Input: part model. Units: mm. Frame: model coordinates. Face numbers are marked on the shaded views. A direction names the side the tool comes from. Coordinates: 2 decimals unless noted, no trailing zeros. Write each loop counter-clockwise with the first axis right and the second up, starting at its lowest first coordinate (ties: lowest second). Pieces come first, ordered by that corner, then holes.
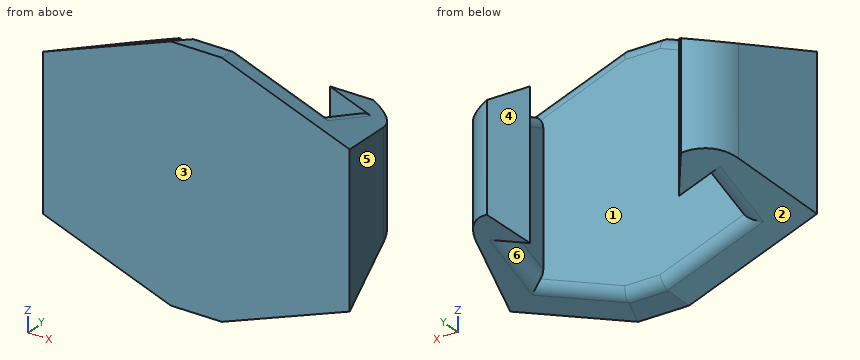
from build123d import *

# Parameters (mm, degrees)
EXTRUDE_1_DEPTH          = 20
CUT_EXTRUDE_1_DEPTH      = 26.52668646
CUT_EXTRUDE_1_DEPTH_BACK = 26.52668646
FILLET_1_R               = 4
CHAMFER_1_SIZE           = 10
CHAMFER_1_SIZE_2         = 3.739269956
FILLET_2_R               = 1


with BuildPart() as part:
    # 草圖2 → 填料-伸長1 (new body)
    with BuildSketch(Plane.XY):
        Polygon((-8.195537152, 3.678491207), (-10.195537152, 3.678491207), (-10.195537152, -0.821508793), (5.804462848, -0.821508793), (5.804462848, 3.678491207), (3.804462848, 3.678491207), (5.618474025, 6.178491207), (7.618474025, 6.178491207), (10.163991353, -3.321508793), (-14.609516351, -3.321508793), (-12.063999023, 6.178491207), (-10.063999023, 6.178491207), align=None)
    extrude(amount=EXTRUDE_1_DEPTH)

    # 草圖3 → 除料-伸長1 (cut, two sides: drawn at the far end of the back side and taken through both)
    with BuildSketch(Plane(origin=(0, 0, 0), x_dir=(0, 0, -1), z_dir=(1, 0, 0)).offset(-CUT_EXTRUDE_1_DEPTH_BACK)):
        Polygon((-20, -3.321508793), (-17.454482672, 6.178491207), (-20, 6.178491207), align=None)
        Polygon((0, 6.178491207), (-2.545517328, 6.178491207), (0, -3.321508793), align=None)
    extrude(amount=CUT_EXTRUDE_1_DEPTH + CUT_EXTRUDE_1_DEPTH_BACK, mode=Mode.SUBTRACT)

    # 圓角1
    # the kernel refuses this fillet: 4 mm, written as the material it takes off along each edge
    with BuildSketch(Plane(origin=(7.618474025, 6.178491207, -4.720017408), x_dir=(-1, 0, 0), z_dir=(0, 0, 1))) as fillet_1_piece_1:
        with BuildLine():
            CenterArc((3.1115198, 3.842463238), FILLET_1_R, 195, 58.866285833)
            Line((-0.752183505, 2.807187057), (-0.829457571, 2.786481534))
            Line((-0.829457571, 2.786481534), (-0.077274066, -0.020705524))
            Line((-0.077274066, -0.020705524), (0, -0.08))
            ThreePointArc((0, -0.08), (1, -0.08), (1.977769604, -0.076849265))
            Line((1.977769604, -0.076849265), (2, 0))
        make_face()
    extrude(amount=29.440034816, mode=Mode.SUBTRACT)
    with BuildSketch(Plane(origin=(-12.063999023, 6.178491207, -4.720017408), x_dir=(1, 0, 0), z_dir=(0, 0, 1))) as fillet_1_piece_2:
        with BuildLine():
            CenterArc((3.1115198, -3.842463238), FILLET_1_R, 106.133714167, 58.866285833)
            Line((-0.752183505, -2.807187057), (-0.829457571, -2.786481534))
            Line((-0.829457571, -2.786481534), (-0.077274066, 0.020705524))
            Line((-0.077274066, 0.020705524), (0, 0.08))
            ThreePointArc((0, 0.08), (1, 0.08), (1.977769604, 0.076849265))
            Line((1.977769604, 0.076849265), (2, 0))
        make_face()
    extrude(amount=29.440034816, mode=Mode.SUBTRACT)

    # 導角1
    # the kernel refuses this chamfer: 10, 3.739269956 mm, written as the material it takes off along each edge
    with BuildSketch(Plane(origin=(16.664078496, -27.580164265, -6.500087143), x_dir=(-0.9680162049238082, -0.23859176587740763, -0.07757961240176374), z_dir=(-0.25056280708573614, 0.9351131265310298, 0.25056280708572526)), Plane(origin=(-6.316095385, 27.629959622, 8.293420966), x_dir=(0.9680162049238085, -0.23859176587740732, -0.0775796124017635), z_dir=(-0.2505628070857358, -0.93511312653103, -0.2505628070857253)), Plane(origin=(-21.109603495, -27.580164265, 26.500087143), x_dir=(0.9680162049238082, -0.23859176587740735, 0.07757961240176349), z_dir=(0.25056280708573586, 0.9351131265310301, -0.2505628070857251)), Plane(origin=(1.870570387, 27.629959622, 11.706579034), x_dir=(-0.9680162049238082, -0.23859176587740777, 0.07757961240176336), z_dir=(0.25056280708573614, -0.93511312653103, 0.25056280708572504))) as chamfer_1_piece_1:
        Polygon((CHAMFER_1_SIZE * 0.999913086528, CHAMFER_1_SIZE * 0.0131840581986), (-CHAMFER_1_SIZE_2 * 0.080135920558, CHAMFER_1_SIZE_2 * 0.996783945724), (0, 0), align=None)
    extrude(amount=59.041117401, mode=Mode.SUBTRACT)

    # 圓角2
    fillet_2_edges = [part.edges().sort_by_distance(p)[0] for p in [
        (5.804462848, 1.428491207, 16.018986119),
        (5.804462848, 1.428491207, 3.981013881),
        (-2.222762499, -0.821508793, 19.330127019),
        (-2.222762499, -0.821508793, 0.669872981),
        (2.484536748, -0.821508793, 18.088717027),
        (-6.902836399, -0.821508793, 18.098897319),
        (-6.902836399, -0.821508793, 1.901102681),
        (2.484536748, -0.821508793, 1.911282973),
        (-10.195537152, 1.428491207, 16.039346704),
        (-10.195537152, 1.428491207, 3.960653296),
    ]]
    fillet(fillet_2_edges, radius=FILLET_2_R)


solid = part.part
Item 1: Pin query (flat end, axial travel): pin 1 Ø5 at (y, z) = (1, 10) entering from -X; pin 2 Ø5 at (y, z) = (0.5, 8.5) entering from +X; pin 3 Ø3 at (y, z) = (-1.5, 12) entering from +X; pin 4 Ø4 at (y, z) = (-1.5, 5.5) entering from -X. Return the tip coordinate at first contact, or that it passes through.
Item 2: Access query for the marked faces 4, 5 and 6. Directions: +Z, -Z, +X, -X, +Y, -Y. A direction counts if a zero-diameter tool reaches every point of the face in a straight line with its end or side. Return the directions, or none.
Item 3: Section query D-D, the plane x = -12.5. Return loops of the section in (y, z).
Item 4: Pull-direction query (Y, two-part tool) for the marked faces 1, 2 and 3; classes: released by +Y, released by -Y, zero draft, split by the parting line, or undercut.
Item 5: Section query B-B, the plane z = 8.5. Return loops of the section in (x, y).
Item 6: Section query C-C, the plane y = -2.25. Return loops of the section in (x, z).
Item 7: Material intervals for line 1 (Y direction, x = -1.75, z = 17); line 2 (Y direction, x = -10, z = 10); line 3 (Y direction, x = 4.25, z = 10.75), sorted ascending.
Item 8: Section query A-A, the plane y = 4.75. Return loops of the section in (x, z).
The answers:
1. pin 1: stops at x = -14.12
1. pin 2: stops at x = 9.81
1. pin 3: stops at x = 10.08
1. pin 4: stops at x = -14.61
2. face 4: +Z, -Z, +Y
2. face 5: +Z, -Z, +X, +Y
2. face 6: -Z
3. outline: (-3.32, 3.07) - (4.18, 5.84) - (4.18, 14.16) - (-3.32, 16.93) - close
4. face 1: undercut
4. face 2: released by +Y
4. face 3: released by -Y
5. outline: (-14.61, -3.32) - (10.16, -3.32) - (8.37, 3.37) arc R4 ccw to (5.62, 6.18) - (3.8, 3.68) - (5.8, 3.68) - (5.8, -0.82) - (-10.2, -0.82) - (-10.2, 3.68) - (-8.2, 3.68) - (-10.06, 6.18) arc R4 ccw to (-12.82, 3.37) - close
6. outline: (-14.32, 4.15) - (-3.99, 0.29) - (-0.45, 0.29) - (9.88, 4.15) - (9.88, 15.85) - (-0.45, 19.71) - (-3.99, 19.71) - (-14.32, 15.85) - close
7. line 1: y = -3.32 to -0.82
7. line 2: y = -3.32 to -0.82, 3.68 to 6.09
7. line 3: y = -3.32 to -0.82, 3.68 to 4.29
8. outline: (-12.14, 5.91) - (-9, 4.74) - (-9, 15.26) - (-12.14, 14.09) - close; (4.58, 4.75) - (7.7, 5.91) - (7.7, 14.09) - (4.58, 15.25) - close
